The model under review builds one solid part; all positions refer to its coordinate system, in mm. A direction names the side the tool comes from. Round coordinates to 2 decimals unless told otherwise and drop trailing zeros. Write each loop counter-clockwise with the first axis right and the second up, starting at its lowest first coordinate (ties: lowest second). Pieces come first, ordered by that corner, then holes. Notation, with made-up numbers: (51, -11) -> (104, -11) arc R35 cw to (104, 21) -> close; hole circle Ø10 at (31, -1). An arc over 180 degrees is marked (long way). Return JSON: item names as keys, results as strings. Group by question number.
1. For line 1 along Y through (x, z) = (6.25, -2.5); line 2 along X through (y, z) = (46, 0); line 3 along Y through (x, z) = (-4, 3.25), list the stretches that pass through material, from the lowest coordinate up. Write a range as from..to.
2. Mouldability with a two-part tool opening along Y and no side actions: class faces 6 (the flat face through (-6, 110.5, 0)), 7 (the flat face through (1, 56, 5)), 8 (the cylindrical face through (9.99, 5.51, -0.44)) as pulls with the +Y half, pulls with the -Y half, needs draft (parallel to the pull), parting line crosses it, or undercut.
3. Tool access review of faces 1 (the flat face through (-4, 56, -1)), 2 (the flat face through (-2, 3, -6)), 3 (the cylindrical face through (9, 56, 0)), 4 (the cylindrical face through (-4.032, 1.521, -6.324)), 5 (the cylindrical face through (0, 56, -9)): name each direction out of +Z, -Z, +X, -X, +Y, -Y from which nothing blocks a thin tool from reaching the whole face with its end or side.
4. Clearance check with flat-ended pins moving along their axes: P1, Ø1, axis at x = 3, y = 71, coming from the -Z side; P2, Ø12, axis at y = 96.5, z = -9.5, coming from the +X side; P3, Ø4, axis at y = 47, z = -9.5, coming from the -X side. State where each tip first meets the part, or that it passes through.
5. Take a section at A-A, the plane y = 40.5. Write out the cut boundary in (x, z), then the cut area to 3 significant figures.
from build123d import *

# Parameters (mm, degrees)
SKETCH4_W           = 2
SKETCH4_H           = 2
BOSS_EXTRUDE5_DEPTH = 102
SKETCH5_R           = 13
BOSS_EXTRUDE6_DEPTH = 2.5
BOSS_EXTRUDE7_DEPTH = 1
FILLET1_R           = 1


with BuildPart() as part:
    # Sketch3 → Revolve1 (revolve)
    with BuildSketch(Plane.XY, mode=Mode.PRIVATE) as revolve1_sk:
        Polygon((0, 0), (7.5, 0), (7.5, 3), (6, 3), (6, 5), (10, 5), (10, 6), (0, 6), align=None)
    revolve(revolve1_sk.sketch.rotate(Axis((0, 6, 0), (0, -1, 0)), 180), axis=Axis((0, 6, 0), (0, -1, 0)))

    # Sketch4 → Boss-Extrude5 (add)
    with BuildSketch(Plane(origin=(0, 6, 0), x_dir=(1, 0, 0), z_dir=(0, 1, 0))):
        with BuildLine():
            ThreePointArc((1, 8), (0, 9), (-1, 8))
            Line((-1, 8), (-1, 1))
            Line((-1, 1), (1, 1))
            Line((1, 1), (1, 8))
        make_face()
        with BuildLine():
            Line((-1, -1), (-1, 1))
            Line((-1, 1), (-8, 1))
            ThreePointArc((-8, 1), (-9, 0), (-8, -1))
            Line((-8, -1), (-1, -1))
        make_face()
        with BuildLine():
            Line((1, -1), (-1, -1))
            Line((-1, -1), (-1, -8))
            ThreePointArc((-1, -8), (0, -9), (1, -8))
            Line((1, -8), (1, -1))
        make_face()
        with BuildLine():
            Line((8, 1), (1, 1))
            Line((1, 1), (1, -1))
            Line((1, -1), (8, -1))
            ThreePointArc((8, -1), (9, 0), (8, 1))
        make_face()
        Rectangle(SKETCH4_W, SKETCH4_H)
    extrude(amount=BOSS_EXTRUDE5_DEPTH)

    # Sketch5 → Boss-Extrude6 (add)
    with BuildSketch(Plane(origin=(0, 108, 0), x_dir=(1, 0, 0), z_dir=(0, 1, 0))):
        with Locations(Location((0, 0, 0), (0, 0, 270))):
            Circle(SKETCH5_R)
    extrude(amount=BOSS_EXTRUDE6_DEPTH)

    # Sketch8 → Boss-Extrude7 (add)
    with BuildSketch(Plane(origin=(0, 110.5, 0), x_dir=(1, 0, 0), z_dir=(0, 1, 0))):
        with BuildLine():
            Line((-1.5, 10), (-1.5, -10))
            ThreePointArc((-1.5, -10), (0, -11.5), (1.5, -10))
            Line((1.5, -10), (1.5, 10))
            ThreePointArc((1.5, 10), (0, 11.5), (-1.5, 10))
        make_face()
        with BuildLine():
            Line((-5.5, 8), (-5.5, -8))
            ThreePointArc((-5.5, -8), (-4, -9.5), (-2.5, -8))
            Line((-2.5, -8), (-2.5, 8))
            ThreePointArc((-2.5, 8), (-4, 9.5), (-5.5, 8))
        make_face()
        with BuildLine():
            Line((-9.5, 6), (-9.5, -6))
            ThreePointArc((-9.5, -6), (-8, -7.5), (-6.5, -6))
            Line((-6.5, -6), (-6.5, 6))
            ThreePointArc((-6.5, 6), (-8, 7.5), (-9.5, 6))
        make_face()
        with BuildLine():
            Line((6.5, 6), (6.5, -6))
            ThreePointArc((6.5, -6), (8, -7.5), (9.5, -6))
            Line((9.5, -6), (9.5, 6))
            ThreePointArc((9.5, 6), (8, 7.5), (6.5, 6))
        make_face()
        with BuildLine():
            Line((5.5, 8), (5.5, -8))
            ThreePointArc((5.5, -8), (4, -9.5), (2.5, -8))
            Line((2.5, -8), (2.5, 8))
            ThreePointArc((2.5, 8), (4, 9.5), (5.5, 8))
        make_face()
    extrude(amount=BOSS_EXTRUDE7_DEPTH)

    # Fillet1
    fillet1_edges = [part.edges().sort_by_distance(p)[0] for p in [
        (9.5, 111.5, 0),
        (8, 111.5, 7.5),
        (6.5, 111.5, 0),
        (8, 111.5, -7.5),
        (5.5, 111.5, 0),
        (4, 111.5, 9.5),
        (2.5, 111.5, 0),
        (4, 111.5, -9.5),
        (1.5, 111.5, 0),
        (0, 111.5, 11.5),
        (-1.5, 111.5, 0),
        (0, 111.5, -11.5),
        (-2.5, 111.5, 0),
        (-4, 111.5, 9.5),
        (-5.5, 111.5, 0),
        (-4, 111.5, -9.5),
        (-6.5, 111.5, 0),
        (-8, 111.5, 7.5),
        (-9.5, 111.5, 0),
        (-8, 111.5, -7.5),
    ]]
    fillet(fillet1_edges, radius=FILLET1_R - 0.0001)  # a hair under: the kernel refuses the full size


solid = part.part
Output:
{
 "1": {"line 1": "y = 0..3, 5..6, 108..110.5", "line 2": "x = -9..9", "line 3": "y = 0..6, 108..111.5"},
 "2": {"face 6": "pulls with the +Y half", "face 7": "undercut", "face 8": "needs draft"},
 "3": {"face 1": "-Z, -X", "face 2": "none", "face 3": "+X", "face 4": "-Y", "face 5": "-Z"},
 "4": {"P1": "stops at z = -1", "P2": "stops at x = 1", "P3": "stops at x = -1"},
 "5": {"outline": "(-8, -1) -> (-1, -1) -> (-1, -8) arc R1 ccw to (1, -8) -> (1, -1) -> (8, -1) arc R1 ccw to (8, 1) -> (1, 1) -> (1, 8) arc R1 ccw to (-1, 8) -> (-1, 1) -> (-8, 1) arc R1 ccw to start", "area": "66.3 mm^2"}
}
